Could you check a few things on this model? Use its own coordinates, in mm. A direction names the side the tool comes from. Give positions to 0.01 mm unless a question says otherwise; leave off trailing zeros. Loops run counter-clockwise (first coordinate to the right, second up) from the corner with the lowest first, then second, coordinate; pieces in that order, holes last.
1. Imagine slicing it at D-D (y = 12). List the corners of the cut face in (x, z) for me, plus the area to 3 significant figures.
2. Imagine slicing it at A-A (z = 39.8). List the corners of the cut face in (x, y) for me.
3. Imagine slicing it at B-B (z = 6). List the corners of the cut face in (x, y) for me.
4. Imagine slicing it at C-C (y = 5). List the corners of the cut face in (x, z) for me.
5. For faces 1 (the flat face through (-14, 4, 4.8)), 2 (the flat face through (-3.504, 10, 28)), 3 (the flat face through (-3.997, 6.716, 27.691)), which set-ups out of +Z, -Z, +X, -X, +Y, -Y let a thin tool reach every point of the face, with its end or its side?
6. I need wall thicknesses on line 1 along Y through (x, z) = (-8, 31); line 2 along X through (y, z) = (0.8, 39.8); line 3 along Y through (x, z) = (-3.25, 39). Which ranges of each line are inside material? Lowest first, please.
7. For P1, Ø3.5, axis at x = -4.5, y = 3, coming from the +Z side; P2, Ø4.5, axis at y = 10.5, z = 22, coming from the +X side; P3, Ø2, axis at x = -11, y = 3, coming from the -Z side; P4, Ø3.5, axis at x = 3.5, y = 8.5, coming from the +Z side, each with a flat end and sliding along its axis, tell me the tip position at first contact or that it passes through.
8. Thinking about a two-plate mould opening in Z: for faces 4 (the cylindrical face through (-7.326, 0.156, 41.191)), 5 (the flat face through (2, 8, 9)), 6 (the flat face through (-21.513, 1, 17)), which applies, +Z half, -Z half, draft (parallel to the pull), parting line (faces both ways), or undercut?
Autodesk Inventor part; units mm, degrees
ref_plane "YZ Plane" through (0, 0, 0) normal (1, 0, 0) x (0, 1, 0)
ref_plane "XZ Plane" through (0, 0, 0) normal (0, 1, 0) x (-1, 0, 0)
ref_plane "XY Plane" through (0, 0, 0) normal (0, 0, 1) x (1, 0, 0)
sketch "Sketch1" plane through (0, 0, 0) normal (0, 0, 1) x (1, 0, 0)
  line L0 (-23.7129, 7.994) -> (-21.7129, 5.994)
  line L1 (-21.7129, 0.4463) -> (-21.7129, 5.994)
  line L2 (-19.7129, -1.5537) -> (-21.7129, 0.4463)
  line L3 (3.2871, -1.5537) -> (-19.7129, -1.5537)
  line L4 (5.2871, 0.4463) -> (3.2871, -1.5537)
  line L5 (5.2871, 5.994) -> (5.2871, 0.4463)
  line L6 (5.2871, 5.994) -> (7.2871, 7.994)
  line L7 (-23.5715, 8.1354) -> (-21.5129, 6.0768)
  line L8 (-21.5129, 6.0768) -> (-21.5129, 0.5292)
  line L9 (-21.5129, 0.5292) -> (-19.6301, -1.3537)
  line L10 (-19.6301, -1.3537) -> (3.2042, -1.3537)
  line L11 (3.2042, -1.3537) -> (5.0871, 0.5292)
  line L12 (5.0871, 0.5292) -> (5.0871, 6.0768)
  line L13 (5.0871, 6.0768) -> (7.1456, 8.1354)
  line L14 (-21.5129, 6.0768) -> (-19.6301, 8.8175)
  line L15 (-19.6301, 8.8175) -> (-11.568, 13.3014)
  line L16 (-11.568, 13.3014) -> (-8.2129, 13.3014)
  line L17 (-19.7129, -1.5537) -> (-19.7129, -4.3475)
  line L18 (-19.7129, -4.3475) -> (-8.2129, -4.3475)
  line L19 (-8.2129, -4.3475) -> (-8.2129, 15.1673)
  line L20 (5.0871, 6.0768) -> (3.2042, 8.8175)
  line L21 (3.2042, 8.8175) -> (-4.8579, 13.3014)
  line L22 (-4.8579, 13.3014) -> (-8.2129, 13.3014)
  point P0 (0, 0)
  dimension "d0" = 0.2
  dimension "d1" = 23
  dimension "d2" = 11.5
extrude "Extrusion1" add sketch "Sketch1" along normal blind 42.8 contours L10 L9 L8 L14 L15 L16 L19 | L19 L22 L21 L20 L12 L11 L10
sketch "Sketch2" plane through (0, 0, 0) normal (0, 0, -1) x (-1, 0, 0)
  line L0 (13.2269, 1.874) -> (13.2269, 5.874)
  line L1 (3.0769, 5.874) -> (13.2269, 5.874)
  line L2 (3.0769, 5.874) -> (3.0769, 1.874)
  line L3 (3.6906, 5.9511) -> (12.5906, 5.9511)
  line L4 (12.5906, 5.9511) -> (12.5906, 1.9511)
  line L5 (12.5906, 1.9511) -> (3.6906, 1.9511)
  line L6 (3.6906, 1.9511) -> (3.6906, 5.9511)
  point P0 (0, 0)
  dimension "d5" = 4
  dimension "d6" = 8.9
extrude "Extrusion2" cut sketch "Sketch2" against normal blind 4.8
sketch "Sketch3" plane through (0, 0, 4.8) normal (0, 0, -1) x (-1, 0, 0)
  line L0 (-8.749, 6.2089) -> (25.106, 6.2089)
  line L1 (25.106, 6.2089) -> (25.106, 1.7089)
  line L2 (25.106, 1.7089) -> (-8.749, 1.7089)
  line L3 (-8.749, 1.7089) -> (-8.749, 6.2089)
  point P0 (0, 0)
  dimension "d9" = 4.5
extrude "Extrusion3" cut sketch "Sketch3" against normal through all
sketch "Sketch4" plane through (-19.6301, -1.3537, 0) normal (0, -1, 0) x (1, 0, 0)
  line L0 (0, 0) -> (0, 42.8)
  line L1 (0, 39.8) -> (11.4172, 39.8)
  line L2 (11.4172, 39.8) -> (22.8343, 39.8)
  line L3 (22.8343, 0) -> (22.8343, 42.8)
  circle A0 centre (11.4172, 39.8) radius 1.65
  line L4 (0, 42.8) -> (22.8343, 42.8)
  point P0 (19.6301, 0)
  dimension "d12" = 3
  dimension "d13" = 3.3
extrude "Extrusion4" cut sketch "Sketch4" against normal through all contours A0 L2 L1 | L1 L2 A0
sketch "Sketch5" plane through (-11.568, 13.3014, 0) normal (0, 1, 0) x (1, 0, 0)
  line L0 (7.8774, 0) -> (7.8774, -4.8)
  line L1 (-1.0226, 0) -> (-1.0226, -4.8)
  line L2 (-1.3542, -46.1873) -> (-11.7813, -46.1873)
  line L3 (-11.7813, -46.1873) -> (-11.7813, -9)
  line L4 (-11.7813, -9) -> (-5.3542, -9)
  line L5 (-1.3542, -13) -> (-1.3542, -46.1873)
  line L6 (8.0643, -44.7269) -> (19.9839, -44.7269)
  line L7 (19.9839, -44.7269) -> (19.9839, -9)
  line L8 (19.9839, -9) -> (12.0643, -9)
  line L9 (8.0643, -13) -> (8.0643, -44.7269)
  line L10 (16.5643, -42.8) -> (16.5643, -4.8)
  line L11 (-9.8542, -4.8) -> (-9.8542, -42.8)
  line L12 (14.7722, 0) -> (6.7101, 0)
  line L13 (12.0643, -9) -> (8.0643, -13)
  line L14 (-1.3542, -13) -> (-5.3542, -9)
  point P0 (11.568, 0)
  point P1 (-1.3542, -9)
  point P2 (8.0643, -9)
  dimension "d16" = 8.5
  dimension "d17" = 8.5
  dimension "d18" = 9
  dimension "d19" = 4
  dimension "d20" = 4
  dimension "d21" = 4
  dimension "d22" = 4
extrude "Extrusion5" cut sketch "Sketch5" against normal up to surface (11.5925 mm away)
chamfer "Chamfer1" distance 1 angle 45 2 edges at (-3.5036, 6.2089, 27.9) (-12.9222, 6.2089, 27.9)
equation "\"d17\" = d16"
properties part number "charge_port_plug"
Derived:
1. outline: (-13.91, 0) - (-2.52, 0) - (-2.52, 12.01) - (-3.5, 13) - (-3.5, 42.8) - (-12.92, 42.8) - (-12.92, 13) - (-13.91, 12.01) - close; hole circle Ø3.3 at (-8.21, 39.8)
1. area: 419 mm2
2. outline: (-21.51, 0.53) - (-19.63, -1.35) - (-9.86, -1.35) - (-9.86, 1.71) - (-21.51, 1.71) - close; (-12.92, 7.21) - (-11.92, 6.21) - (-9.86, 6.21) - (-9.86, 13.3) - (-11.57, 13.3) - (-12.92, 12.55) - close; (-6.56, -1.35) - (3.2, -1.35) - (5.09, 0.53) - (5.09, 1.71) - (-6.56, 1.71) - close; (-6.56, 6.21) - (-4.5, 6.21) - (-3.5, 7.21) - (-3.5, 12.55) - (-4.86, 13.3) - (-6.56, 13.3) - close
3. outline: (-21.51, 0.53) - (-19.63, -1.35) - (3.2, -1.35) - (5.09, 0.53) - (5.09, 1.71) - (-21.51, 1.71) - close; (-21.42, 6.21) - (5, 6.21) - (3.2, 8.82) - (-4.86, 13.3) - (-11.57, 13.3) - (-19.63, 8.82) - close
4. outline: (-21.51, 0) - (-12.59, 0) - (-12.59, 4.8) - (-21.51, 4.8) - close; (-3.69, 0) - (5.09, 0) - (5.09, 4.8) - (-3.69, 4.8) - close
5. face 1: +Z, +X, -X
5. face 2: +Z, +X, +Y
5. face 3: +Z, +X
6. line 1: y = -1.35 to 1.71, 6.21 to 13.3
6. line 2: x = -21.51 to -9.86, -6.56 to 5.09
6. line 3: y = -1.35 to 1.71
7. P1: stops at z = 42.8
7. P2: stops at x = -3.5
7. P3: passes through
7. P4: stops at z = 9
8. face 4: undercut
8. face 5: +Z half
8. face 6: draft
